from build123d import *

# Parameters (mm, degrees)
F1_DEPTH = 7.5


with BuildPart() as f1:
    # F0 (on Top) → F1 (new body)
    with BuildSketch(Plane.XY):
        with BuildLine():
            ThreePointArc((4.055896, -5.191311), (4.334412, -5.34336), (4.636016, -5.244746))
            ThreePointArc((4.636016, -5.244746), (6.707186, 2.003412), (1, 6.928203))
            Line((1, 6.928203), (1, 14.928203))
            ThreePointArc((1, 14.928203), (0, 17.546237), (-1, 14.928203))
            Line((-1, 14.928203), (-1, 6.928203))
            ThreePointArc((-1, 6.928203), (-6.707186, 2.003412), (-4.636016, -5.244746))
            ThreePointArc((-4.636016, -5.244746), (-4.334412, -5.34336), (-4.055896, -5.191311))
            Line((-4.055896, -5.191311), (-3.989942, -5.106893))
            ThreePointArc((-3.989942, -5.106893), (-3.885697, -4.757275), (-4.046721, -4.429904))
            ThreePointArc((-4.046721, -4.429904), (0, 6), (4.046721, -4.429904))
            ThreePointArc((4.046721, -4.429904), (3.885697, -4.757275), (3.989942, -5.106893))
            Line((3.989942, -5.106893), (4.055896, -5.191311))
        make_face()
    extrude(amount=F1_DEPTH)


solid = f1.part
Can you work these out from the model? Positions are in its coordinate system, mm. A direction names the side the tool comes from. Give positions to 0.01 mm unless a question says otherwise; leave off trailing zeros. Loops run counter-clockwise (first coordinate to the right, second up) from the corner with the lowest first, then second, coordinate; pieces in that order, holes last. Notation, with made-up numbers: (-15, 38) - (24, 38) arc R18 cw to (24, 44) - close; hole circle Ø1 at (-18, -13.5). An arc over 180 degrees is marked (long way). Answer as a JSON object with one key per item and string values.
Q1. If I drill on L1, parallel to X at y = 0, z = 2; L2, parallel to X at y = 10.75, z = 2; L3, parallel to Y at x = -4.75, z = 5.75, over which ranges is the centre line in solid material (lowest first)?
Geometry says:
{"L1": "-7 to -6, 6 to 7", "L2": "-1 to 1", "L3": "-5.14 to -3.67, 3.67 to 5.14"}
Q2. Imagine slicing it at D-D on y = 8. Write out the boundary of the cut face in (x, z), plus the area to 3 significant figures.
Geometry says:
{"outline": "(-1, 0) - (1, 0) - (1, 7.5) - (-1, 7.5) - close", "area": "15.0 mm²"}
Q3. Imagine slicing it at A-A on y = 0. Write out the boundary of the cut face in (x, z), plus the area to 3 significant figures.
Geometry says:
{"outline": "(-7, 0) - (-6, 0) - (-6, 7.5) - (-7, 7.5) - close; (6, 0) - (7, 0) - (7, 7.5) - (6, 7.5) - close", "area": "15.0 mm²"}
Q4. If we mould it in two halves opening along Y, with no side actions, what happens to faces 4 (the cylindrical face through (0.051, 17.545, 3.698)), 5 (the flat face through (0, 6.2, 7.5))? For each: pulls with the +Y half, pulls with the -Y half, needs draft (parallel to the pull), parting line crosses it, or undercut.
Geometry says:
{"face 4": "undercut", "face 5": "needs draft"}
Q5. Imagine slicing it at B-B on z = 4. Write out the boundary of the cut face in (x, y), plus the area to 3 significant figures.
Geometry says:
{"outline": "(-4.64, -5.24) arc R0.4 ccw to (-4.06, -5.19) - (-3.99, -5.11) arc R0.5 ccw to (-4.05, -4.43) arc R6 cw (long way) to (4.05, -4.43) arc R0.5 ccw to (3.99, -5.11) - (4.06, -5.19) arc R0.4 ccw to (4.64, -5.24) arc R7 ccw to (1, 6.93) - (1, 14.93) arc R1.5 ccw (long way) to (-1, 14.93) - (-1, 6.93) arc R7 ccw to start", "area": "54.5 mm²"}
Q6. Imagine slicing it at C-C on x = 1.25. Write out the boundary of the cut face in (y, z), plus the area to 3 significant figures.
Geometry says:
{"outline": "(5.87, 0) - (6.89, 0) - (6.89, 7.5) - (5.87, 7.5) - close; (15.22, 0) - (16.88, 0) - (16.88, 7.5) - (15.22, 7.5) - close", "area": "20.1 mm²"}
Q7. Will these pins go through, and if not, where does the flat tip stop? P1, Ø7, axis at x = 0, y = 0, coming from the -Z side; P2, Ø1.5, axis at y = 9, z = 5, coming from the +X side; P3, Ø3, axis at x = 4, z = 4.5, coming from the +Y side.
Geometry says:
{"P1": "through", "P2": "x = 1", "P3": "y = 6.54"}
Q8. Which directions (+Z, -Z, +X, -X, +Y, -Y) give clear straight access to the entire face, cutting with the end or side of a thin tool? Please do faces 1 (the flat face through (1, 11, 4)), 2 (the cylindrical face through (0, 6, 4)), 3 (the flat face through (-1, 11, 4)).
Geometry says:
{"face 1": "+Z, -Z, +X", "face 2": "+Z, -Z", "face 3": "+Z, -Z, -X"}
